Autodesk Inventor part; units mm, degrees
ref_plane "Work Plane1" through (-4, 0, 0) normal (1, 0, 0) x (0, 1, 0)
ref_plane "XZ Plane" through (0, 0, 0) normal (0, 1, 0) x (-1, 0, 0)
ref_plane "XY Plane" through (0, 0, 0) normal (0, 0, 1) x (1, 0, 0)
sketch "Sketch1" plane through (0, 0, 0) normal (0, 1, 0) x (-1, 0, 0)
  arc A0 (3.873, 1) -> (3.873, -1) centre (0, 0) ccw
  circle A1 centre (0, 0) radius 4
  dimension "d0" = 8
extrude "Extrusion1" add sketch "Sketch1" along normal blind 56.5
sketch "Sketch2" plane through (0, 0, 0) normal (1, 0, 0) x (0, 1, 0)
  line L0 (1.5, -6.5) -> (2.44, -6.5)
  line L1 (2.44, -6.5) -> (2.44, -3.5)
  line L2 (2.44, -3.5) -> (1.5, -3.5)
  line L3 (1.5, -3.5) -> (1.5, -6.5)
  line L4 (0, -4) -> (56.5, -4)
  line L5 (0, -4) -> (56.5, -4)
  line L6 (0, -4) -> (56.5, -4)
  line L7 (0, -4) -> (0, 4)
  line L8 (28.25, -4) -> (28.25, 9.3026)
  line L9 (55, -6.5) -> (54.06, -6.5)
  line L10 (54.06, -6.5) -> (54.06, -3.5)
  line L11 (54.06, -3.5) -> (55, -3.5)
  line L12 (55, -3.5) -> (55, -6.5)
  line L13 (56.5, -4) -> (56.5, 4)
  line L14 (-11.3, 0) -> (67.8, 0)
  point P0 (0, 0)
  point P1 (0, 1)
  point P2 (0, -1)
  point P3 (56.5, 0)
  point P4 (56.5, 1)
  point P5 (56.5, -1)
  dimension "d9" = 0.94
  dimension "d10" = 0.5
  dimension "d11" = 3
  dimension "d12" = 1.5
revolve "Revolution1" cut sketch "Sketch2" angle 360 about axis through (0, -10, 0) along (0, 1, 0) contours L3 L4 L1 L0 | L3 L2 L1 L4 | L10 L11 L12 L4 | L4 L12 L9 L10
ref_plane "Work Plane1" through (-4, 0, 0) normal (1, 0, 0) x (0, 1, 0)
sketch "Sketch5" plane through (-4, 0, 0) normal (1, 0, 0) x (0, 1, 0)
  line L0 (42.5, 1) -> (24.5, 1)
  line L1 (24.5, 1) -> (24.5, -1)
  line L2 (24.5, -1) -> (42.5, -1)
  line L3 (42.5, -1) -> (42.5, 1)
  circle A0 centre (24.5, 0) radius 1
  circle A1 centre (42.5, 0) radius 1
  line L4 (2.44, -4) -> (54.06, -4)
  line L5 (2.44, 4) -> (54.06, 4)
  line L6 (56.5, -4) -> (56.5, 4)
  line L7 (0, 4) -> (0, -4)
  point P0 (0, 0)
  dimension "d19" = 2
  dimension "d20" = 3
  dimension "d23" = 18
  dimension "d25" = 14
extrude "Extrusion4" cut sketch "Sketch5" along normal blind 1.2
properties part number "AxeVerticalCaptif" material "Stainless Steel"
Check sheet for the modelled part. Datum: model origin and axes. Units: mm. A direction names the side the tool comes from. Round coordinates to 2 decimals unless told otherwise and drop trailing zeros. Write each loop counter-clockwise with the first axis right and the second up, starting at its lowest first coordinate (ties: lowest second). Pieces come first, ordered by that corner, then holes. Notation, with made-up numbers: M 48,-26.75 L 77,-26.75 A8 cw 77,-21.75 Z; hole C 44.25,-20 d9. An arc over 180 degrees is marked long. Write item = value, one per line. Start each with the question number.
1. Section check D-D, the plane x = -1. Record the cut outline in (y, z).
2. Section check A-A, the plane z = 0. Record the cut outline in (x, y).
3. Tool access check on faces 5 (the cylindrical face through (1.341, 54.537, -3.233)), 6 (the cylindrical face through (-4, 56, 0)), 7 (the flat face through (-3, 34, 1)). Record the directions out of +Z, -Z, +X, -X, +Y, -Y that give a thin tool (end or side, any length) a straight path to the whole face; none if there is none.
4. Scan lines: line 1 (Y direction, x = 2.25, z = 3.25); line 2 (X direction, y = 44, z = 0.25); line 3 (Z direction, x = -2, y = 13). Record each from-to range of solid material in increasing order. Write a range as [from, to].
5. Section check C-C, the plane y = 27. Record the cut outline in (x, z), then the cut area to 4 significant figures.
6. Release check for a two-part mould opening along Y. For faces 1 (the cylindrical face through (4, 1, 0)), 2 (the flat face through (0, 56.5, 0)), 3 (the flat face through (0, 0, 0)), 4 (the cylindrical face through (-3.4, 43.5, 0)) record: pulls with the +Y half, pulls with the -Y half, needs draft (parallel to the pull), parting line crosses it, or undercut.
7. Gauge pin test, flat ends, axial feed: pin 1 (1.2 mm diameter, centred on x = -3.5, y = 32, fed in from +Z) (3 decimals); pin 2 (0.6 mm diameter, centred on y = 33.5, z = 0, fed in from -X). Record the tip position at first contact, or that the pin passes through.
8. Section check B-B, the plane x = 2.75. Record the cut outline in (y, z), then the cut area to 3 significant figures.
Results found:
q1.outline = M 0,-3.87 L 1.5,-3.87 L 1.5,-3.35 L 2.44,-3.35 L 2.44,-3.87 L 54.06,-3.87 L 54.06,-3.35 L 55,-3.35 L 55,-3.87 L 56.5,-3.87 L 56.5,3.87 L 55,3.87 L 55,3.35 L 54.06,3.35 L 54.06,3.87 L 2.44,3.87 L 2.44,3.35 L 1.5,3.35 L 1.5,3.87 L 0,3.87 Z
q2.outline = M -4,0 L 4,0 L 4,1.5 L 3.5,1.5 L 3.5,2.44 L 4,2.44 L 4,54.06 L 3.5,54.06 L 3.5,55 L 4,55 L 4,56.5 L -4,56.5 L -4,55 L -3.5,55 L -3.5,54.06 L -4,54.06 L -4,43.5 L -2.8,43.5 L -2.8,23.5 L -4,23.5 L -4,2.44 L -3.5,2.44 L -3.5,1.5 L -4,1.5 Z
q3.face_5 = none
q3.face_6 = -X, +Y, -Y
q3.face_7 = -X
q4.line_1 = [0, 1.5], [2.44, 54.06], [55, 56.5]
q4.line_2 = [-3.99, 3.99]
q4.line_3 = [-3.46, 3.46]
q5.outline = M -3.87,-1 A4 ccw long -3.87,1 L -2.8,1 L -2.8,-1 Z
q5.area = 47.95 mm^2
q6.face_1 = needs draft
q6.face_2 = pulls with the +Y half
q6.face_3 = pulls with the -Y half
q6.face_4 = undercut
q7.pin_1 = 2.755
q7.pin_2 = -2.8
q8.outline = M 0,-2.9 L 1.5,-2.9 L 1.5,-2.17 L 2.44,-2.17 L 2.44,-2.9 L 54.06,-2.9 L 54.06,-2.17 L 55,-2.17 L 55,-2.9 L 56.5,-2.9 L 56.5,2.9 L 55,2.9 L 55,2.17 L 54.06,2.17 L 54.06,2.9 L 2.44,2.9 L 2.44,2.17 L 1.5,2.17 L 1.5,2.9 L 0,2.9 Z
q8.area = 325 mm^2
